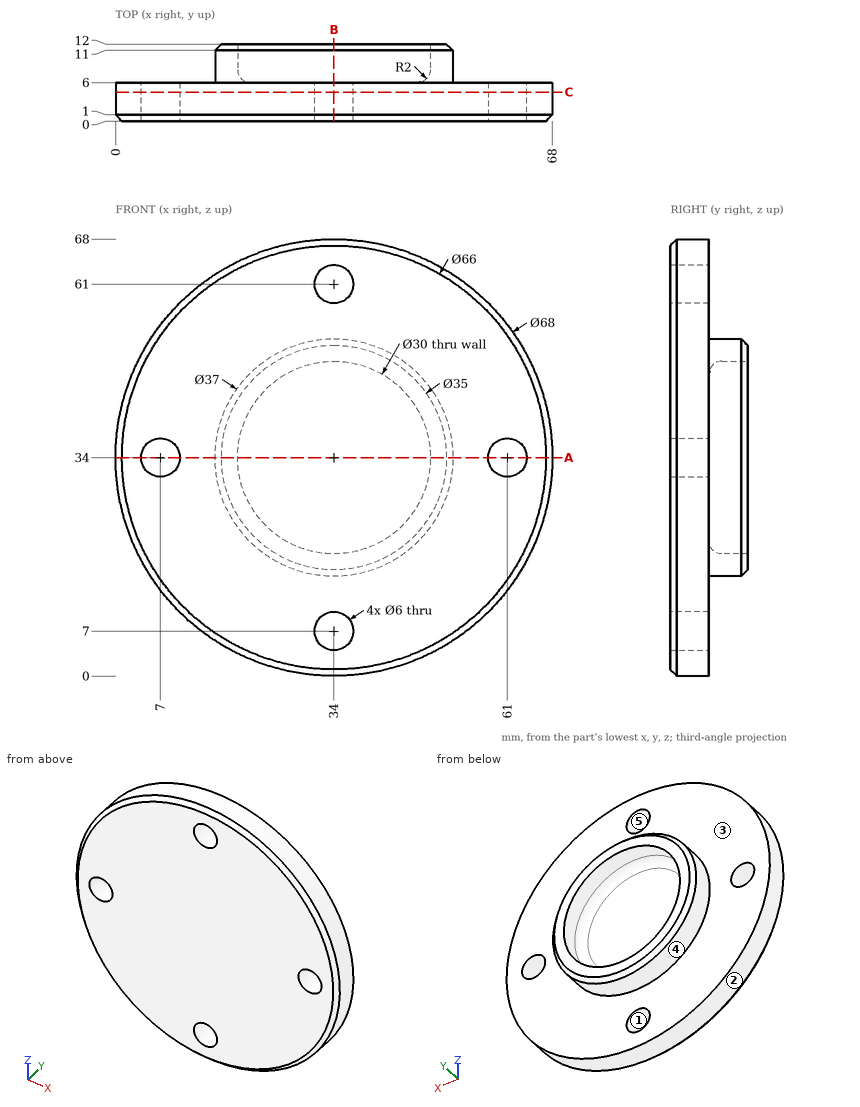
Geometry: see drawing. Coordinates: mm, zero at the bounding-box minimum. A direction names the side the tool comes from. Give positions to 0.01 mm unless a question says otherwise; leave off trailing zeros. Write each loop counter-clockwise with the first axis right and the second up, starting at its lowest first coordinate (ties: lowest second). Pieces come first, ordered by that corner, then holes. Notation, with made-up numbers: (69, 64.25) - (98, 64.25) arc R21 cw to (98, 88.25) - close; hole circle Ø8 at (-9, -16). An arc over 180 degrees is marked (long way). Return JSON: item names as keys, results as strings. Group by question number.
1) Mould query, pull axis Z, two halves, no side actions, for the marked faces 1, 2 and 3. Classes: released by +Z, released by -Z, zero draft, split by the parting line, or undercut.
2) Set-up query: the marked faces 4 and 5. Return all of +Z, -Z, +X, -X, +Y, -Y with unobstructed straight access to the full face (end or side cutting, diameter ignored); none if empty.
3) Section B-B on x = 34. Return the cut outline in (y, z).
4) Section A-A on z = 34. Return the cut outline in (x, y), plus the area to 3 significant figures.
5) Section C-C on y = 4.5. Return the cut outline in (x, z).
6) Line query: line 1 (X direction, y = 2.25, z = 32); line 2 (X direction, y = 4.25, z = 36.5); line 3 (Y direction, x = 24, z = 14.5). Output: solid intervals per line, ascending.
7) First-contact query: P1, Ø6, axis at x = 9.5, z = 9.5, coming from the -Y side; P2, Ø9.5, axis at x = 34, z = 61, coming from the +Y side; P3, Ø5, axis at x = 15, y = 10.5, coming from the +Z side; P4, Ø3.5, axis at x = 7, z = 34, coming from the +Y side. Flat tips, straight axial feed; report the tip coordinate or a pass-through.
Filled in:
{
 "1": {"face 1": "undercut", "face 2": "split by the parting line", "face 3": "zero draft"},
 "2": {"face 4": "+Y", "face 5": "+Y, -Y"},
 "3": {"outline": "(0, 1) - (1, 0) - (6, 0) - (6, 4) - (0, 4) - close; (0, 10) - (6, 10) - (6, 15.5) - (11, 15.5) - (12, 16.5) - (12, 19) - (8, 19) arc R2 cw to (6, 21) - (6, 47) arc R2 cw to (8, 49) - (12, 49) - (12, 51.5) - (11, 52.5) - (6, 52.5) - (6, 58) - (0, 58) - close; (0, 64) - (6, 64) - (6, 68) - (1, 68) - (0, 67) - close"},
 "4": {"outline": "(0, 1) - (1, 0) - (4, 0) - (4, 6) - (0, 6) - close; (10, 0) - (58, 0) - (58, 6) - (52.5, 6) - (52.5, 11) - (51.5, 12) - (49, 12) - (49, 8) arc R2 cw to (47, 6) - (21, 6) arc R2 cw to (19, 8) - (19, 12) - (16.5, 12) - (15.5, 11) - (15.5, 6) - (10, 6) - close; (64, 0) - (67, 0) - (68, 1) - (68, 6) - (64, 6) - close", "area": "378 mm^2"},
 "5": {"outline": "circle Ø68 at (34, 34); hole circle Ø6 at (7, 34); hole circle Ø6 at (34, 7); hole circle Ø6 at (34, 61); hole circle Ø6 at (61, 34)"},
 "6": {"line 1": "x = 0.06 to 4.76, 9.24 to 58.76, 63.24 to 67.94", "line 2": "x = 0.09 to 5.34, 8.66 to 59.34, 62.66 to 67.91", "line 3": "y = 0 to 6"},
 "7": {"P1": "stops at y = 0", "P2": "stops at y = 6", "P3": "stops at z = 42.37", "P4": "passes through"}
}
